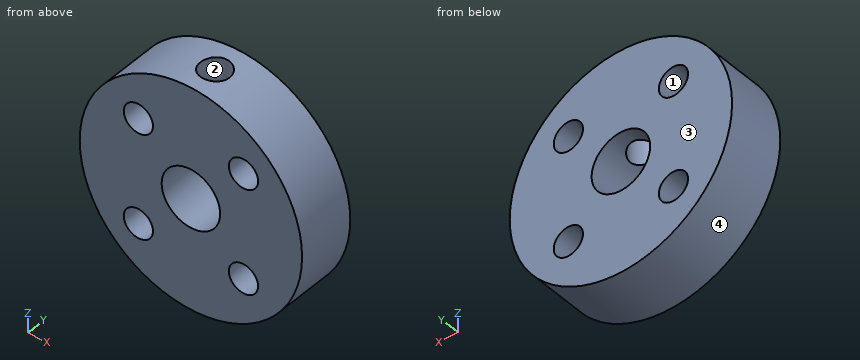
from build123d import *

# Parameters (mm, degrees)
SKETCH1_R                 = 9.5
BOSS_EXTRUDE1_DEPTH       = 5
F_5_0MM_DOWEL_HOLE1_D     = 5
M3X0_5_TAPPED_HOLE1_D     = 2.5
M3X0_5_TAPPED_HOLE2_D     = 2.5
M3X0_5_TAPPED_HOLE2_DEPTH = 10
M3X0_5_TAPPED_HOLE2_TIP   = 0.751075774


with BuildPart() as part:
    # Sketch1 → Boss-Extrude1 (new body)
    with BuildSketch(Plane(origin=(0, 0, 0), x_dir=(1, 0, 0), z_dir=(0, 1, 0))):
        Circle(SKETCH1_R)
    extrude(amount=BOSS_EXTRUDE1_DEPTH)

    # Ø5.0mm Dowel Hole1 (through all)
    with Locations(Plane(origin=(0, 5, 0), x_dir=(1, 0, 0), z_dir=(0, 1, 0))):
        with Locations((0, 0)):
            Hole(F_5_0MM_DOWEL_HOLE1_D / 2)

    # M3x0.5 Tapped Hole1 (through all)
    with Locations(Plane(origin=(0, 5, 0), x_dir=(1, 0, 0), z_dir=(0, 1, 0))):
        with Locations((4.490128061, 4.490128061), (-4.490128061, 4.490128061), (-4.490128061, -4.490128061), (4.490128061, -4.490128061)):
            Hole(M3X0_5_TAPPED_HOLE1_D / 2)

    # M3x0.5 Tapped Hole2
    with Locations(Plane(origin=(0, 2.5, 9.5), x_dir=(1, 0, 0), z_dir=(0, 0, 1))):
        with Locations((0, 0)):
            Hole(M3X0_5_TAPPED_HOLE2_D / 2, depth=M3X0_5_TAPPED_HOLE2_DEPTH)
            with Locations((0, 0, -(M3X0_5_TAPPED_HOLE2_DEPTH + M3X0_5_TAPPED_HOLE2_TIP / 2))):  # 118° drill point
                Cone(0, M3X0_5_TAPPED_HOLE2_D / 2, M3X0_5_TAPPED_HOLE2_TIP, mode=Mode.SUBTRACT)


solid = part.part
Model file for the job. Use its own axes, mm. Face numbers are marked on the shaded views. Give positions to 0.01 mm unless a question says otherwise; leave off trailing zeros. Loops run counter-clockwise (first coordinate to the right, second up) from the corner with the lowest first, then second, coordinate; pieces in that order, holes last. Notation, with made-up numbers: (-27, 34.5) -> (12, 34.5) arc R30 ccw to (12, 62.5) -> close; hole circle Ø3 at (56, 20.25). An arc over 180 degrees is marked (long way). Use a Markdown table: item, result. Add a question column.
(1) Slice it at C-C on z = -4. List the corners of the cut face in (x, y), and give its area (3 significant figures).
(2) Mould opens along X. For the marked faces 1, 2, 3 and 4 say: +X half, -X half, draft (parallel to the pull), parting line (faces both ways), or undercut.
(3) Drop flat-ended pins along their axis: pin 1 Ø1.5 at (y, z) = (2.5, 2) entering from +X; pin 2 Ø3 at (x, z) = (-4.49, -4.49) entering from -Y; pin 3 Ø1 at (y, z) = (0.5, -5.5) entering from -X; pin 4 Ø2 at (x, z) = (-0.5, -0.5) entering from +Y. Give the stop position or say it passes through.
(4) Slice it at A-A on x = 0. List the corners of the cut face in (y, z).
(5) Slice it at B-B on y = 2.5. List the corners of the cut face in (x, z).
(6) Slice it at D-D on y = 0.85. List the corners of the cut face in (x, z).
(7) Wall check: line 1 along Z through (x, y) = (3.5, 0.55); line 2 along X through (y, z) = (2.6, -4); line 3 along Z through (x, y) = (-4.5, 4.55). Give the ranges that are in metal, low to high.
Filled sheet:
| question | item | result |
|---|---|---|
| 1 | outline | (-8.62, 0) -> (-5.64, 0) -> (-5.64, 5) -> (-8.62, 5) -> close; (-3.34, 0) -> (3.34, 0) -> (3.34, 5) -> (-3.34, 5) -> close; (5.64, 0) -> (8.62, 0) -> (8.62, 5) -> (5.64, 5) -> close |
| 1 | area | 63.2 mm2 |
| 2 | face 1 | undercut |
| 2 | face 2 | undercut |
| 2 | face 3 | draft |
| 2 | face 4 | parting line |
| 3 | pin 1 | x = 9.42 |
| 3 | pin 2 | y = 0 |
| 3 | pin 3 | x = -8.08 |
| 3 | pin 4 | through |
| 4 | outline | (0, -9.5) -> (5, -9.5) -> (5, -2.5) -> (0, -2.5) -> close; (0, 2.5) -> (1.25, 2.5) -> (1.25, 9.5) -> (0, 9.5) -> close; (3.75, 2.5) -> (5, 2.5) -> (5, 9.5) -> (3.75, 9.5) -> close |
| 5 | outline | (-1.25, 2.17) -> (-1.25, 9.42) arc R9.5 ccw (long way) to (1.25, 9.42) -> (1.25, 2.17) arc R2.5 cw (long way) to start; hole circle Ø2.5 at (-4.49, -4.49); hole circle Ø2.5 at (-4.49, 4.49); hole circle Ø2.5 at (4.49, -4.49); hole circle Ø2.5 at (4.49, 4.49) |
| 6 | outline | circle Ø19 at (0, 0); hole circle Ø2.5 at (-4.49, -4.49); hole circle Ø2.5 at (-4.49, 4.49); hole circle Ø5 at (0, 0); hole circle Ø2.5 at (4.49, -4.49); hole circle Ø2.5 at (4.49, 4.49) |
| 7 | line 1 | -8.83 to -5.25, -3.73 to 3.73, 5.25 to 8.83 |
| 7 | line 2 | -8.62 to -5.64, -3.34 to 3.34, 5.64 to 8.62 |
| 7 | line 3 | -8.37 to -5.74, -3.24 to 3.24, 5.74 to 8.37 |
